from build123d import *

# Parameters (mm, degrees)
SKETCH_1_R          = 20
EXTRUDE_1_DEPTH     = 8
SKETCH_3_R          = 11
EXTRUDE_2_DEPTH     = 35
CUT_EXTRUDE_1_DEPTH = 46
SKETCH_6_R          = 2.4
CUT_EXTRUDE_2_DEPTH = 44.011626335
SKETCH_7_R          = 6.65
CUT_EXTRUDE_3_DEPTH = 44.011626335


with BuildPart() as part:
    # 草图1 → 凸台-拉伸1 (new body)
    with BuildSketch(Plane(origin=(0, 0, 0), x_dir=(1, 0, 0), z_dir=(0, 1, 0))):
        with Locations(Location((0, 0, 0), (0, 0, 270))):
            Circle(SKETCH_1_R)
    extrude(amount=EXTRUDE_1_DEPTH)

    # 草图3 → 凸台-拉伸2 (add)
    with BuildSketch(Plane.XZ):
        with Locations(Location((0, 0, 0), (0, 0, 270))):
            Circle(SKETCH_3_R)
    extrude(amount=-EXTRUDE_2_DEPTH)

    # 草图4 → 切除-拉伸1 (cut, through all)
    with BuildSketch(Plane.XZ):
        with BuildLine():
            Line((-15, 13.228756555), (-15, -13.228756555))
            ThreePointArc((-15, -13.228756555), (-20, 0), (-15, 13.228756555))
        make_face()
        with BuildLine():
            Line((15, 13.228756555), (15, -13.228756555))
            ThreePointArc((15, -13.228756555), (20, 0), (15, 13.228756555))
        make_face()
    extrude(amount=-CUT_EXTRUDE_1_DEPTH, mode=Mode.SUBTRACT)

    # 草图6 → 切除-拉伸2 (cut, through all)
    with BuildSketch(Plane.XZ):
        with Locations(Location((0, 16, 0), (0, 0, 270))):
            Circle(SKETCH_6_R)
        with Locations(Location((11.313708499, 11.313708499, 0), (0, 0, 270))):
            Circle(SKETCH_6_R)
        with Locations(Location((11.313708499, -11.313708499, 0), (0, 0, 270))):
            Circle(SKETCH_6_R)
        with Locations(Location((0, -16, 0), (0, 0, 270))):
            Circle(SKETCH_6_R)
        with Locations(Location((-11.313708499, -11.313708499, 0), (0, 0, 270))):
            Circle(SKETCH_6_R)
        with Locations(Location((-11.313708499, 11.313708499, 0), (0, 0, 270))):
            Circle(SKETCH_6_R)
    extrude(amount=-CUT_EXTRUDE_2_DEPTH, mode=Mode.SUBTRACT)

    # 草图7 → 切除-拉伸3 (cut, through all)
    with BuildSketch(Plane.XZ):
        with Locations(Location((0, 0, 0), (0, 0, 270))):
            Circle(SKETCH_7_R)
    extrude(amount=-CUT_EXTRUDE_3_DEPTH, mode=Mode.SUBTRACT)


solid = part.part
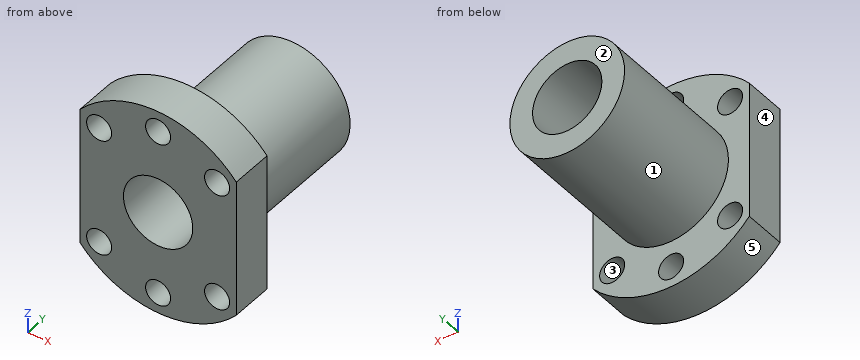
Design review of the part built by this model. Coordinates are the model's own, in mm. Face numbers are marked on the shaded views. A direction names the side the tool comes from. Round coordinates to 2 decimals unless told otherwise and drop trailing zeros. Write each loop counter-clockwise with the first axis right and the second up, starting at its lowest first coordinate (ties: lowest second). Pieces come first, ordered by that corner, then holes. Notation, with made-up numbers: M 88.25,-21 L 145.25,-21 A14 cw 145.25,-5 Z; hole C -1.5,68 d5. An arc over 180 degrees is marked long. One line per item, written item: value. Start each with the question number.
1. For the marked faces 1 and 2, list the 3-axis set-ups (+Z, -Z, +X, -X, +Y, -Y) from which the entire face can be reached by the end or side of a thin tool; tool diameter is ignored.
2. Draft analysis for pull direction X (two halves, no side actions). For the marked faces 3, 4 and 5, state which applies: pulls with the +X half, pulls with the -X half, needs draft (parallel to the pull), parting line crosses it, or undercut.
3. To check wall thickness, follow probe 1 along X at (y, z) = (11, 0); probe 2 along X at (y, z) = (5, -16); probe 3 along Z at (x, y) = (4, 21). State the ranges of each line that lie inside material, in increasing order. Write a range as from..to.
4. Take a section at D-D on y = 27.5. State the section outline as (x, z) points.
5. Take a section at B-B on x = 0. State the section outline as (y, z) points, then the cut area to 3 significant figures.
6. Take a section at A-A on z = -16. State the section outline as (x, y) points, then the cut area to 3 significant figures.
7. Clearance check with flat-ended pins moving along their axes: P1, Ø4, axis at x = -9.5, z = -11, coming from the -Y side; P2, Ø3, axis at x = 0, z = -16, coming from the -Y side; P3, Ø6, axis at y = 24.5, z = 13, coming from the +X side; P4, Ø12, axis at y = 27, z = -8, coming from the +X side. State where each tip first meets the part, or that it passes through.
8. Take a section at C-C on y = 6.5. State the section outline as (x, z) points, then the cut area to 3 significant figures.
Computed:
1. face 1: +Y
1. face 2: +Z, -Z, +X, -X, +Y
2. face 3: undercut
2. face 4: pulls with the -X half
2. face 5: parting line crosses it
3. probe 1: x = -11..-6.65, 6.65..11
3. probe 2: x = -12..-2.4, 2.4..12
3. probe 3: z = -10.25..-5.31, 5.31..10.25
4. outline: C 0,0 d22; hole C 0,0 d13.3
5. outline: M 0,-20 L 8,-20 L 8,-18.4 L 0,-18.4 Z; M 0,-13.6 L 8,-13.6 L 8,-11 L 35,-11 L 35,-6.65 L 0,-6.65 Z; M 0,6.65 L 35,6.65 L 35,11 L 8,11 L 8,13.6 L 0,13.6 Z; M 0,18.4 L 8,18.4 L 8,20 L 0,20 Z
5. area: 372 mm²
6. outline: M -12,0 L -2.4,0 L -2.4,8 L -12,8 Z; M 2.4,0 L 12,0 L 12,8 L 2.4,8 Z
6. area: 154 mm²
7. P1: stops at y = 0
7. P2: passes through
7. P3: stops at x = 4.58
7. P4: stops at x = 10.82
8. outline: M -15,-13.23 A20 ccw 15,-13.23 L 15,13.23 A20 ccw -15,13.23 Z; hole C -11.31,-11.31 d4.8; hole C -11.31,11.31 d4.8; hole C 0,0 d13.3; hole C 0,-16 d4.8; hole C 0,16 d4.8; hole C 11.31,-11.31 d4.8; hole C 11.31,11.31 d4.8
8. area: 828 mm²
